Verification items for the finished model (mm, model axes). Face numbers are marked on the shaded views. A direction names the side the tool comes from. Round coordinates to 2 decimals unless told otherwise and drop trailing zeros. Order: outer loops, then holes, each group sorted by start corner. A loop starts at its lowest first (then second) coordinate and runs counter-clockwise, first axis right, second up. Notation, with made-up numbers: M 63,16 L 92,16 A26 ccw 92,41 Z; hole C -38.5,-31 d10. An arc over 180 degrees is marked long. One line per item, written item: value. Start each with the question number.
from build123d import *

# Parameters (mm, degrees)
SKETCH1_W           = 4
SKETCH1_H           = 5.75
SKETCH1_W_2         = 2
SKETCH1_H_2         = 2.5
SKETCH1_W_3         = 2.25
BOSS_EXTRUDE1_DEPTH = 8.75
FILLET1_R           = 0.9
SKETCH2_W           = 2
SKETCH2_H           = 10.75
BOSS_EXTRUDE2_DEPTH = 10
CUT_EXTRUDE1_DEPTH  = 13.5
FILLET2_R           = 4.5


with BuildPart() as part:
    # Sketch1 → Boss-Extrude1 (new body)
    with BuildSketch(Plane(origin=(0, 0, 0), x_dir=(1, 0, 0), z_dir=(0, 1, 0))):
        with Locations((-6.25, 0)):
            Rectangle(SKETCH1_W, SKETCH1_H)
        with Locations((-3.25, 4.125)):
            Rectangle(SKETCH1_W_2, SKETCH1_H_2)
        with Locations((-3.25, -4.125)):
            Rectangle(SKETCH1_W_2, SKETCH1_H_2)
        with Locations((-3.25, 0)):
            Rectangle(SKETCH1_W_2, SKETCH1_H)
        with Locations((-1.125, 0)):
            Rectangle(SKETCH1_W_3, SKETCH1_H)
        with Locations((1.125, 0)):
            Rectangle(SKETCH1_W_3, SKETCH1_H)
        with Locations((3.25, 4.125)):
            Rectangle(SKETCH1_W_2, SKETCH1_H_2)
        with Locations((6.25, 0)):
            Rectangle(SKETCH1_W, SKETCH1_H)
        with Locations((3.25, 0)):
            Rectangle(SKETCH1_W_2, SKETCH1_H)
        with Locations((3.25, -4.125)):
            Rectangle(SKETCH1_W_2, SKETCH1_H_2)
    extrude(amount=BOSS_EXTRUDE1_DEPTH)

    # Fillet1
    fillet1_edges = [part.edges().sort_by_distance(p)[0] for p in [
        (-8.25, 4.375, 2.875),
        (-8.25, 4.375, -2.875),
        (8.25, 4.375, -2.875),
        (8.25, 4.375, 2.875),
    ]]
    fillet(fillet1_edges, radius=FILLET1_R)

    # Sketch2 → Boss-Extrude2 (add)
    with BuildSketch(Plane(origin=(0, 8.75, 0), x_dir=(1, 0, 0), z_dir=(0, 1, 0))):
        with Locations((-3.25, 0)):
            Rectangle(SKETCH2_W, SKETCH2_H)
    extrude(amount=BOSS_EXTRUDE2_DEPTH)

    # Sketch3 → Cut-Extrude1 (cut, through all)
    with BuildSketch(Plane.ZY.offset(4.25)):
        Polygon((-5.375, 18.75), (-5.375, 15.031688137), (-4.097886003, 18.75), align=None)
        Polygon((-2.273593829, 18.75), (-4.097886003, 18.75), (-3.185739916, 14.925754612), align=None)
        Polygon((1.282681443, 18.75), (-2.273593829, 18.75), (-0.495456193, 15.243564513), align=None)
        Polygon((4.097886003, 18.75), (1.282681443, 18.75), (2.690283723, 15.079098327), align=None)
        Polygon((5.375, 18.75), (4.097886003, 18.75), (5.375, 15.031688137), align=None)
    extrude(amount=-CUT_EXTRUDE1_DEPTH, mode=Mode.SUBTRACT)

    # Fillet2
    fillet2_edges = [part.edges().sort_by_distance(p)[0] for p in [
        (-2.25, 8.75, 0),
    ]]
    fillet(fillet2_edges, radius=FILLET2_R)


solid = part.part
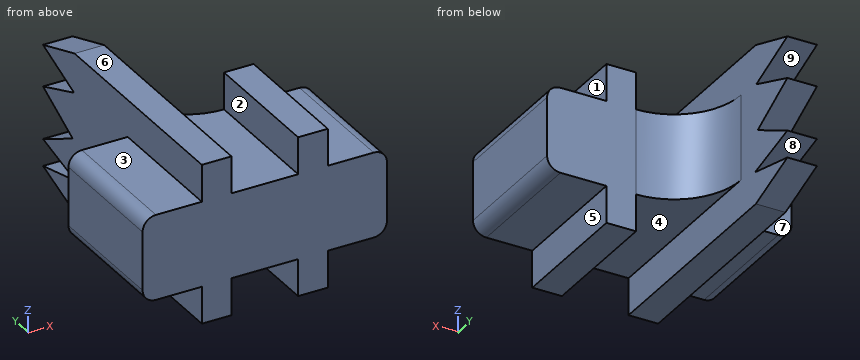
1. Section check B-B (y = 2). Record the cut outline in (x, z) (3 decimals), and give its area (3 significant figures).
2. Tool access check on the marked faces 1, 2, 3, 4 and 5. Record the directions out of +Z, -Z, +X, -X, +Y, -Y that give a thin tool (end or side, any length) a straight path to the whole face; none if there is none.
3. Section check D-D (y = 16.75). Record the cut outline in (x, z).
4. Section check C-C (z = 4.75). Record the cut outline in (x, y).
5. Section check A-A (x = -3.25). Record the cut outline in (y, z) (3 decimals), and give its area (3 significant figures).
6. Draft check along Z on the marked faces 6, 7, 8 and 9. Enter one of: released by +Z, released by -Z, zero draft, split by the parting line, or undercut.
7. Scan lines: line 1 along X through (y, z) = (5, -4.5); line 2 along Z through (x, y) = (-1.25, 7.5) (3 decimals); line 3 along X through (y, z) = (17.25, -4). Record each from-to range of solid material in increasing order.
8. Depth check by flat-ended pin: pin 1 (8 mm diameter, centred on x = 0, y = 13.5, fed in from +Z) (3 decimals); pin 2 (3 mm diameter, centred on y = 6.5, z = 4, fed in from +X); pin 3 (2.5 mm diameter, centred on x = -6, y = 6, fed in from +Z) (3 decimals); pin 4 (2 mm diameter, centred on y = 5, z = -4, fed in from -X). Enter the tip coordinate at first touch or a pass-through.
Geometry check:
1. outline: M -8.25,-1.975 A0.9 ccw -7.35,-2.875 L -4.25,-2.875 L -4.25,-5.375 L -2.25,-5.375 L -2.25,-2.875 L 2.25,-2.875 L 2.25,-5.375 L 4.25,-5.375 L 4.25,-2.875 L 7.35,-2.875 A0.9 ccw 8.25,-1.975 L 8.25,1.975 A0.9 ccw 7.35,2.875 L 4.25,2.875 L 4.25,5.375 L 2.25,5.375 L 2.25,2.875 L -2.25,2.875 L -2.25,5.375 L -4.25,5.375 L -4.25,2.875 L -7.35,2.875 A0.9 ccw -8.25,1.975 Z
1. area: 114 mm²
2. face 1: +Z, +X, +Y, -Y
2. face 2: +Z, +Y, -Y
2. face 3: +Z, -X, +Y, -Y
2. face 4: -Z, +Y, -Y
2. face 5: -Z, +X, +Y, -Y
3. outline: M -4.25,-4.78 L -2.25,-4.78 L -2.25,-3.62 L -4.25,-3.62 Z; M -4.25,-2.75 L -2.25,-2.75 L -2.25,-1.26 L -4.25,-1.26 Z; M -4.25,0.27 L -2.25,0.27 L -2.25,2.05 L -4.25,2.05 Z; M -4.25,3.33 L -2.25,3.33 L -2.25,4.78 L -4.25,4.78 Z
4. outline: M -4.25,0 L -2.25,0 L -2.25,16.85 L -4.25,16.85 Z; M 2.25,0 L 4.25,0 L 4.25,8.75 L 2.25,8.75 Z
5. outline: M 0,-5.375 L 15.032,-5.375 L 18.75,-4.098 L 14.926,-3.186 L 18.75,-2.274 L 15.244,-0.495 L 18.75,1.283 L 15.079,2.69 L 18.75,4.098 L 15.032,5.375 L 0,5.375 Z
5. area: 182 mm²
6. face 6: released by +Z
6. face 7: zero draft
6. face 8: undercut
6. face 9: undercut
7. line 1: x = -4.25 to -2.25, 2.25 to 4.25
7. line 2: z = -2.875 to 2.875
7. line 3: x = -4.25 to -2.25
8. pin 1: stops at z = 5.375
8. pin 2: stops at x = 8.08
8. pin 3: stops at z = 2.875
8. pin 4: stops at x = -4.25
